Part model, mm, in its own coordinate system. A direction names the side the tool comes from. Coordinates: 2 decimals unless noted, no trailing zeros. Order: outer loops, then holes, each group sorted by start corner. A loop starts at its lowest first (then second) coordinate and runs counter-clockwise, first axis right, second up. Notation, with made-up numbers: M -1,-10.75 L 21,-10.75 A17 cw 21,-0.75 Z; hole C -21.5,47.25 d4. An arc over 180 degrees is marked long. Answer in a Markdown table with one row per item. Add a question column.
from build123d import *

# Parameters (mm, degrees)
F1_DEPTH = 15
F2_SIZE2 = 6
F2_SIZE  = 1
F3_W     = 0.66
F3_H     = 0.66
F4_DEPTH = 6.5
F5_R     = 1


with BuildPart() as f1:
    # F0 (on Top) → F1 (new body)
    with BuildSketch(Plane.XY):
        with BuildLine():
            Line((42.301387, 28.022311), (-8.698613, 28.022311))
            ThreePointArc((-8.698613, 28.022311), (-9.46174, 11.022311), (-8.698613, -5.977689))
            Line((-8.698613, -5.977689), (42.301387, -5.977689))
            Line((42.301387, -5.977689), (42.301387, 28.022311))
        make_face()
    extrude(amount=F1_DEPTH)

    # F2
    f2_edges = [f1.edges().sort_by_distance(p)[0] for p in [
        (42.301387, 11.022311, 15),
    ]]
    chamfer(f2_edges, length=F2_SIZE, length2=F2_SIZE2)

    # F3 (on face) → F4 (cut)
    with BuildSketch(Plane.YZ.offset(42.301387)):
        Polygon((9.922311, 12), (-4.077689, 12), (-4.077689, 4.4), (9.922311, 4.4), (10.272311, 4.4), (10.272311, 12), align=None)
        with Locations((-2.747689, 6.17)):
            Rectangle(F3_W, F3_H, mode=Mode.SUBTRACT)
        with Locations((-0.247689, 6.17)):
            Rectangle(F3_W, F3_H, mode=Mode.SUBTRACT)
        with Locations((2.252311, 6.17)):
            Rectangle(F3_W, F3_H, mode=Mode.SUBTRACT)
        with Locations((4.752311, 6.17)):
            Rectangle(F3_W, F3_H, mode=Mode.SUBTRACT)
        with Locations((7.252311, 6.17)):
            Rectangle(F3_W, F3_H, mode=Mode.SUBTRACT)
        with Locations((-2.747689, 8.17)):
            Rectangle(F3_W, F3_H, mode=Mode.SUBTRACT)
        with Locations((-0.247689, 8.17)):
            Rectangle(F3_W, F3_H, mode=Mode.SUBTRACT)
        with Locations((2.252311, 8.17)):
            Rectangle(F3_W, F3_H, mode=Mode.SUBTRACT)
        with Locations((4.752311, 8.17)):
            Rectangle(F3_W, F3_H, mode=Mode.SUBTRACT)
        with Locations((7.252311, 8.17)):
            Rectangle(F3_W, F3_H, mode=Mode.SUBTRACT)
        with Locations((-2.747689, 10.17)):
            Rectangle(F3_W, F3_H, mode=Mode.SUBTRACT)
        with Locations((-0.247689, 10.17)):
            Rectangle(F3_W, F3_H, mode=Mode.SUBTRACT)
        with Locations((2.252311, 10.17)):
            Rectangle(F3_W, F3_H, mode=Mode.SUBTRACT)
        with Locations((4.752311, 10.17)):
            Rectangle(F3_W, F3_H, mode=Mode.SUBTRACT)
        with Locations((7.252311, 10.17)):
            Rectangle(F3_W, F3_H, mode=Mode.SUBTRACT)
        Polygon((12.122311, 12), (11.772311, 12), (11.772311, 4.4), (12.122311, 4.4), (26.122311, 4.4), (26.122311, 12), align=None)
        with Locations((14.792311, 6.17)):
            Rectangle(F3_W, F3_H, mode=Mode.SUBTRACT)
        with Locations((17.292311, 6.17)):
            Rectangle(F3_W, F3_H, mode=Mode.SUBTRACT)
        with Locations((19.792311, 6.17)):
            Rectangle(F3_W, F3_H, mode=Mode.SUBTRACT)
        with Locations((22.292311, 6.17)):
            Rectangle(F3_W, F3_H, mode=Mode.SUBTRACT)
        with Locations((24.792311, 6.17)):
            Rectangle(F3_W, F3_H, mode=Mode.SUBTRACT)
        with Locations((14.792311, 8.17)):
            Rectangle(F3_W, F3_H, mode=Mode.SUBTRACT)
        with Locations((17.292311, 8.17)):
            Rectangle(F3_W, F3_H, mode=Mode.SUBTRACT)
        with Locations((19.792311, 8.17)):
            Rectangle(F3_W, F3_H, mode=Mode.SUBTRACT)
        with Locations((22.292311, 8.17)):
            Rectangle(F3_W, F3_H, mode=Mode.SUBTRACT)
        with Locations((24.792311, 8.17)):
            Rectangle(F3_W, F3_H, mode=Mode.SUBTRACT)
        with Locations((14.792311, 10.17)):
            Rectangle(F3_W, F3_H, mode=Mode.SUBTRACT)
        with Locations((17.292311, 10.17)):
            Rectangle(F3_W, F3_H, mode=Mode.SUBTRACT)
        with Locations((19.792311, 10.17)):
            Rectangle(F3_W, F3_H, mode=Mode.SUBTRACT)
        with Locations((22.292311, 10.17)):
            Rectangle(F3_W, F3_H, mode=Mode.SUBTRACT)
        with Locations((24.792311, 10.17)):
            Rectangle(F3_W, F3_H, mode=Mode.SUBTRACT)
    extrude(amount=-F4_DEPTH, mode=Mode.SUBTRACT)

    # F5
    f5_edges = [f1.edges().sort_by_distance(p)[0] for p in [
        (-8.698613, -5.977689, 7.5),
        (-8.698613, 28.022311, 7.5),
    ]]
    fillet(f5_edges, radius=F5_R)


solid = f1.part
(1) Drop flat-ended pins along their axis: P1, Ø1, axis at y = 4.5, z = 6, coming from the -X side; P2, Ø0.7, axis at x = 38, y = -0.5, coming from the +Z side. Give the stop position or say it passes through.
(2) 3-axis set-ups, long thin cutter, end or side, ignore diameter. For faces 5 (the flat face through (39, 26.122, 8)), 6 (the flat face through (18, 28.022, 7)): which of +Z, -Z, +X, -X, +Y, -Y reach the whole face in a straight line?
(3) Slice it at B-B (z = 9.25). List the corners of the cut face in (x, y), and give its area (3 significant figures).
(4) Slice it at A-A (x = 37). State how many separate pieces and enclosed holes the cut face has, and give its area (3 significant figures).
(5) Slice it at C-C (y = 13). List the corners of the cut face in (x, z), and give its area (3 significant figures).
(6) Slice it at D-D (y = -1.5). List the corners of the cut face in (x, z).
(7) Pull direction Y, two halves, no side cores. Call faces 1 (the flat face through (39, 19, 4.4)), 2 (the flat face through (17, -5.978, 7)), 3 (the cylindrical face through (-8, 28, 8)), 4 (the flat face through (39.3, 10.8, 14.5)): pulls with the +Y half, pulls with the -Y half, needs draft (parallel to the pull), parting line crosses it, or undercut.
(8) Wall check: line 1 (Y direction, x = 38, z = 6.75); line 2 (Z direction, x = 39.5, y = -0.5); line 3 (Z direction, x = 36, y = 16.5). Give the ranges that are in metal, low to high.
Computed:
| question | item | result |
|---|---|---|
| 1 | P1 | stops at x = -9.37 |
| 1 | P2 | stops at z = 14.78 |
| 2 | face 5 | +X |
| 2 | face 6 | +Z, -Z, +X, -X, +Y |
| 3 | outline | M -8.78,-5.06 A1 ccw -7.78,-5.98 L 42.3,-5.98 L 42.3,-4.08 L 35.8,-4.08 L 35.8,10.27 L 42.3,10.27 L 42.3,11.77 L 35.8,11.77 L 35.8,26.12 L 42.3,26.12 L 42.3,28.02 L -7.78,28.02 A1 ccw -8.78,27.11 A189.73 ccw Z |
| 3 | area | 1,560 mm^2 |
| 4 | separate pieces | 31 |
| 4 | enclosed holes | 2 |
| 4 | area | 301 mm^2 |
| 5 | outline | M -9.45,0 L 42.3,0 L 42.3,4.4 L 35.8,4.4 L 35.8,12 L 42.3,12 L 42.3,14 L 36.3,15 L -9.45,15 Z |
| 5 | area | 724 mm^2 |
| 6 | outline | M -9.05,0 L 42.3,0 L 42.3,4.4 L 35.8,4.4 L 35.8,12 L 42.3,12 L 42.3,14 L 36.3,15 L -9.05,15 Z |
| 7 | face 1 | undercut |
| 7 | face 2 | pulls with the -Y half |
| 7 | face 3 | pulls with the +Y half |
| 7 | face 4 | needs draft |
| 8 | line 1 | y = -5.98 to -4.08, 10.27 to 11.77, 26.12 to 28.02 |
| 8 | line 2 | z = 0 to 4.4, 5.84 to 6.5, 7.84 to 8.5, 9.84 to 10.5, 12 to 14.47 |
| 8 | line 3 | z = 0 to 4.4, 12 to 15 |
